Drawing for the job (mm, zero at the part's lowest x, y, z). Coordinates: 2 decimals unless noted, no trailing zeros. Write each loop counter-clockwise with the first axis right and the second up, starting at its lowest first coordinate (ties: lowest second). Pieces come first, ordered by that corner, then holes. Notation, with made-up numbers: (80, -13) -> (109, -13) arc R18 cw to (109, 7) -> close; hole circle Ø3 at (33.25, 38). An arc over 180 degrees is marked (long way). Write item = value, one per line. Start each with the question number.
Q1. Pin check, flat tips, straight feed: P1, Ø6, axis at x = 13.5, z = 22.5, coming from the -Y side; P2, Ø1.1, axis at y = 4.5, z = 21, coming from the +X side (1 decimal); P3, Ø1, axis at y = 3, z = 8.5, coming from the +X side (1 decimal). Stop position of each tip, or through.
Q2. Pull direction Z, two halves, no side cores. Call the marked faces 1, 2 and 3: released by +Z, released by -Z, zero draft, split by the parting line, or undercut.
Q3. Band-saw the part on C-C, the plane y = 3.55. List the corners of the cut face in (x, z).
Q4. Probe line 1 (X direction, y = 4.6, z = 6.5); line 2 (X direction, y = 3.05, z = 11.5) (1 decimal); line 3 (Z direction, x = 13, y = 2.05) (1 decimal). List the from-to ranges inside material, lowest first.
Q5. Band-saw the part on A-A, the plane x = 13. List the corners of the cut face in (y, z).
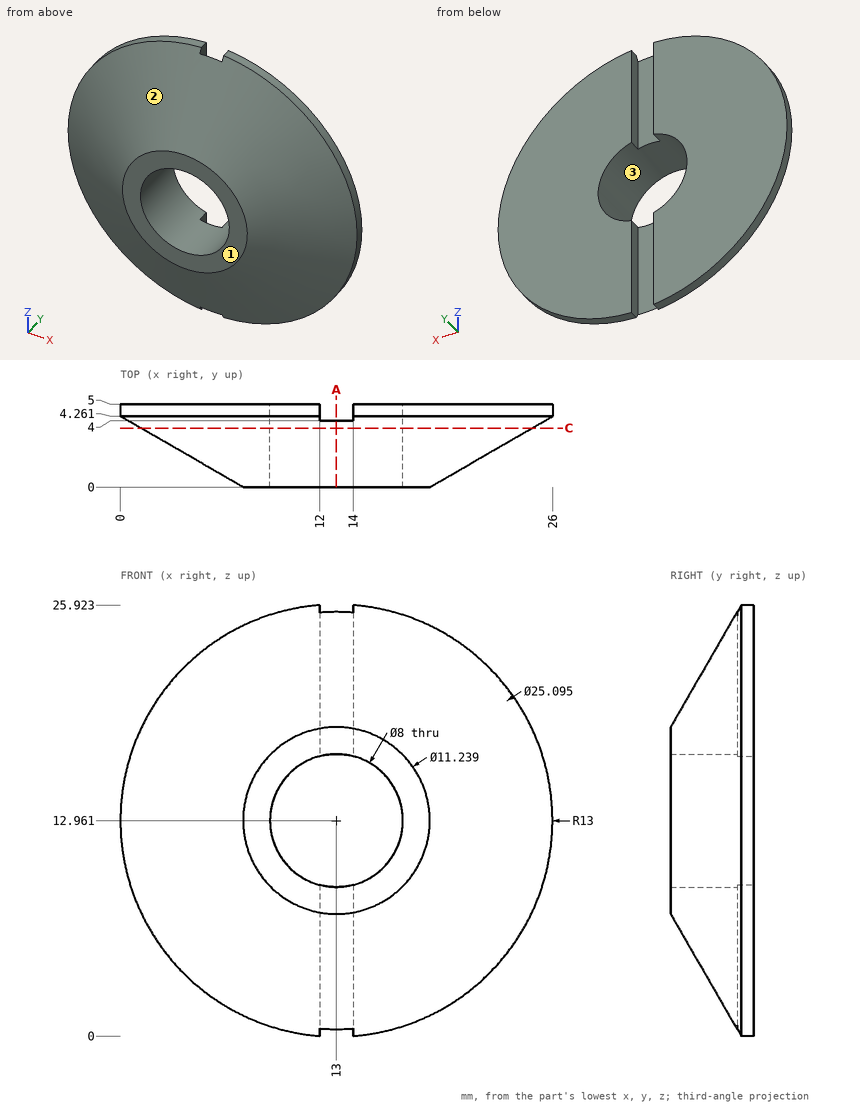
Ans:
q1.P1 = 0.54
q1.P2 = 23.6
q1.P3 = 23.8
q2.face_1 = zero draft
q2.face_2 = split by the parting line
q2.face_3 = undercut
q3.outline = circle Ø23.54 at (13, 12.96); hole circle Ø8 at (13, 12.96)
q4.line_1 = 1.72 to 12, 14 to 24.28
q4.line_2 = 2.2 to 9.3, 16.7 to 23.8
q4.line_3 = 3.8 to 9, 17 to 22.1
q5.outline = (0, 7.34) -> (4, 0.41) -> (4, 8.96) -> (0, 8.96) -> close; (0, 16.96) -> (4, 16.96) -> (4, 25.51) -> (0, 18.58) -> close
